Study the drawing (mm; zero at the part's minimum x, y, z) and answer. Round coordinates to 2 decimals unless told otherwise and drop trailing zeros. Write each loop counter-clockwise with the first axis right and the second up, starting at its lowest first coordinate (ties: lowest second). Pieces come first, ordered by that corner, then holes. Notation, with made-up numbers: M 24.25,39 L 47.25,39 A9 ccw 47.25,44 Z; hole C 48.5,-21 d7. An arc over 180 degrees is marked long. Write each question's results on one line, items separated by ' | '.
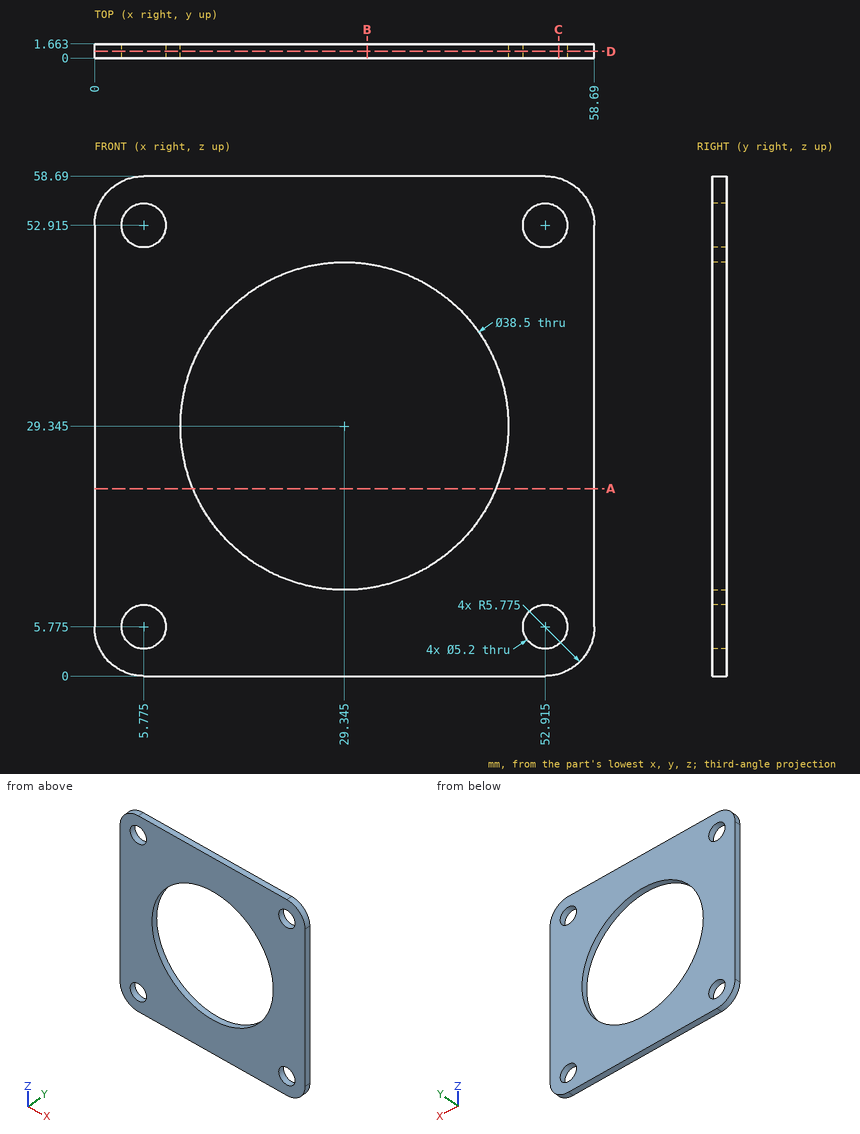
1) Section C-C (x = 54.5) is taken. Determine the outline of the cut face in (y, z).
Return value:
outline: M 0,0.22 L 1.66,0.22 L 1.66,3.71 L 0,3.71 Z; M 0,7.84 L 1.66,7.84 L 1.66,50.85 L 0,50.85 Z; M 0,54.98 L 1.66,54.98 L 1.66,58.47 L 0,58.47 Z
2) Section B-B (x = 32) is taken. Determine the outline of the cut face in (y, z).
Return value:
outline: M 0,0 L 1.66,0 L 1.66,10.28 L 0,10.28 Z; M 0,48.41 L 1.66,48.41 L 1.66,58.69 L 0,58.69 Z
3) Find the intervals of material crossed by line 1 (Z direction, x = 6, y = 1.5) (1 decimal); line 2 (Z direction, x = 29, y = 1.5); line 3 (X direction, y = 0.85, z = 51.5) (1 decimal), in increasing order.
Return value:
line 1: 0 to 3.2, 8.4 to 50.3, 55.5 to 58.7 | line 2: 0 to 10.1, 48.59 to 58.69 | line 3: 0 to 3.6, 8 to 50.7, 55.1 to 58.7
4) Section D-D (y = 0.8) is taken. State how many separate pieces and enclosed holes the cut face has, then the cut area to 3 significant figures.
Return value:
separate pieces: 1 | enclosed holes: 5 | area: 2,170 mm²
5) Section A-A (z = 22) is taken. Determine the outline of the cut face in (x, y).
Return value:
outline: M 0,0 L 11.55,0 L 11.55,1.66 L 0,1.66 Z; M 47.14,0 L 58.69,0 L 58.69,1.66 L 47.14,1.66 Z
